Check sheet for the modelled part. Datum: model origin and axes. Units: mm. Round coordinates to 2 decimals unless told otherwise and drop trailing zeros. Loops run counter-clockwise (first coordinate to the right, second up) from the corner with the lowest first, then second, coordinate; pieces in that order, holes last. Notation, with made-up numbers: (60.5, 17.5) - (99.5, 17.5) arc R13 ccw to (99.5, 29.5) - close; hole circle Ø11 at (-35, -18.75). An arc over 180 degrees is marked (long way). Answer in a Markdown table with one row per item. Add a question column.
(1) Cross-section at B-B on z = -70. Enter the section's corners in (x, y).
(2) Cross-section at A-A on x = 58. Enter the section's corners in (y, z), then the cut area to 3 significant figures.
(3) Thickness scan on line 1 along Z through (x, y) = (120, 1.1); line 2 along X through (y, z) = (0.75, -20); line 3 along X through (y, z) = (0.9, -70). Record the ranges inside material, lowest first.
(4) Mould release check, pull along Z, two halves, no side actions. Record for faces 1 (the flat face through (71, 1, -140)), 2 (the flat face through (71, 0, -69)), 3 (the cylindrical face through (21.08, 1.48, -15.12)): +Z half, -Z half, draft (parallel to the pull), parting line (faces both ways), or undercut.
(5) Cross-section at C-C on x = 120. Enter the section's corners in (y, z).
(6) Cross-section at D-D on y = 0.7. Enter the section's corners in (x, z), then the cut area to 3 significant figures.
(7) Gauge pin test, flat end, axial feed: pin 1 (8 mm diameter, centred on x = 20, z = -20, fed in from -Y). Record the tip position at first contact, or that the pin passes through.
Autodesk Inventor part; units mm, degrees
ref_plane "YZ Plane" through (0, 0, 0) normal (1, 0, 0) x (0, 1, 0)
ref_plane "XZ Plane" through (0, 0, 0) normal (0, 1, 0) x (-1, 0, 0)
ref_plane "XY Plane" through (0, 0, 0) normal (0, 0, 1) x (1, 0, 0)
sketch "Эскиз1" plane through (0, 0, 0) normal (0, 1, 0) x (-1, 0, 0)
  line L0 (0, 0) -> (-140, 0)
  line L1 (-140, 0) -> (-140, -140)
  line L2 (-140, -140) -> (0, -140)
  line L3 (0, -140) -> (0, 0)
  line L4 (0, 0) -> (-20, 0)
  line L5 (-20, 0) -> (-20, -20)
  line L6 (-20, -20) -> (0, -20)
  line L7 (0, -20) -> (0, 0)
  line L8 (-140, -140) -> (-120, -140)
  line L9 (-120, -140) -> (-120, -120)
  line L10 (-120, -120) -> (-140, -120)
  line L11 (-140, -120) -> (-140, -140)
  line L12 (-120, -120) -> (-20, -120)
  line L13 (-20, -120) -> (-20, -20)
  line L14 (-20, -20) -> (-120, -20)
  line L15 (-120, -20) -> (-120, -120)
  circle A0 centre (-20, -20) radius 5
  circle A1 centre (-20, -120) radius 5
  circle A2 centre (-120, -20) radius 5
  circle A3 centre (-120, -120) radius 5
  line L16 (-140, -70) -> (0, -70)
  line L17 (-70, -70) -> (-58, -70)
  line L18 (-58, -70) -> (-82, -70)
  circle A4 centre (-58, -70) radius 3.5
  circle A5 centre (-82, -70) radius 3.5
  dimension "d0" = 140
  dimension "d1" = 140
  dimension "d2" = 20
  dimension "d3" = 20
  dimension "d4" = 20
  dimension "d5" = 20
  dimension "d6" = 10
  dimension "d7" = 10
  dimension "d8" = 10
  dimension "d9" = 10
  dimension "d10" = 12
  dimension "d11" = 24
  dimension "d12" = 7
  dimension "d13" = 7
extrude "Выдавливание1" add sketch "Эскиз1" along normal blind 3 contours L3 L6 A0 L5 L0 | L5 A0 L14 A2 L15 L16 L1 L0 | L3 L16 L13 A0 L6 | L3 L2 L9 A3 L12 A1 L13 L16 | L16 L15 A3 L10 L1 | A0 L13 L16 A4 A5 L15 A2 L14 | L13 A1 L12 A3 L15 L16 A5 A4 | L10 A3 L9 L2 L1
properties part number "Пластина"
Answers:
| question | item | result |
|---|---|---|
| 1 | outline | (0, 0) - (54.5, 0) - (54.5, 3) - (0, 3) - close; (61.5, 0) - (78.5, 0) - (78.5, 3) - (61.5, 3) - close; (85.5, 0) - (140, 0) - (140, 3) - (85.5, 3) - close |
| 2 | outline | (0, -140) - (3, -140) - (3, -73.5) - (0, -73.5) - close; (0, -66.5) - (3, -66.5) - (3, 0) - (0, 0) - close |
| 2 | area | 399 mm^2 |
| 3 | line 1 | z = -140 to -125, -115 to -25, -15 to 0 |
| 3 | line 2 | x = 0 to 15, 25 to 115, 125 to 140 |
| 3 | line 3 | x = 0 to 54.5, 61.5 to 78.5, 85.5 to 140 |
| 4 | face 1 | -Z half |
| 4 | face 2 | draft |
| 4 | face 3 | undercut |
| 5 | outline | (0, -140) - (3, -140) - (3, -125) - (0, -125) - close; (0, -115) - (3, -115) - (3, -25) - (0, -25) - close; (0, -15) - (3, -15) - (3, 0) - (0, 0) - close |
| 6 | outline | (0, -140) - (140, -140) - (140, 0) - (0, 0) - close; hole circle Ø10 at (20, -120); hole circle Ø10 at (20, -20); hole circle Ø7 at (58, -70); hole circle Ø7 at (82, -70); hole circle Ø10 at (120, -120); hole circle Ø10 at (120, -20) |
| 6 | area | 19,200 mm^2 |
| 7 | pin 1 | passes through |
